Geometry check sheet. Reference: the model listing, model coordinates, mm. Face numbers are marked on the shaded views. A direction names the side the tool comes from. Give positions to 0.01 mm unless a question says otherwise; leave off trailing zeros. Loops run counter-clockwise (first coordinate to the right, second up) from the corner with the lowest first, then second, coordinate; pieces in that order, holes last. Notation, with made-up numbers: (16, -30.5) -> (35, -30.5) arc R22 ccw to (35, -13.5) -> close; hole circle Ø8 at (76, 73.5). An arc over 180 degrees is marked (long way). Write each question's results on one line, items separated by ' | '. Start each with the question number.
1) Scan lines: line 1 (Z direction, x = -30, y = -27.5); line 2 (Y direction, x = 2, z = 14); line 3 (Z direction, x = 26, y = -40.5). Record each from-to range of solid material in increasing order. Write a range as from..to.
2) Sectioned sample at B-B on x = 0. Record the cut outline in (y, z).
3) Depth check by flat-ended pin: pin 1 (4 mm diameter, centred on x = -23.81, z = 30.03, fed in from -Y); pin 2 (13.5 mm diameter, centred on x = -13.5, z = 31.5, fed in from +Y); pin 3 (8 mm diameter, centred on y = 6, z = 5, fed in from +X). Enter the tip coordinate at first touch or a pass-through.
4) Sectioned sample at D-D on z = 21.5. Record the cut outline in (x, y).
5) Sectioned sample at A-A on y = 12. Record the cut outline in (x, z), then the cut area to 3 significant figures.
6) Set-up check for the marked faces 1 and 2: record each of +Z, -Z, +X, -X, +Y, -Y from which the full face is reachable in a straight line by a thin tool's end or side.
7) Sectioned sample at C-C on y = -2.5. Record the cut outline in (x, z).
8) Draft check along X on the marked faces 3, 4 and 5. Enter one of: pulls with the +X half, pulls with the -X half, needs draft (parallel to the pull), parting line crosses it, or undercut.
```python
from build123d import *

# Parameters (mm, degrees)
F1_DEPTH = 13
F2_DEPTH = 40
F4_D     = 7


with BuildPart() as f1:
    # F0 (on Top) → F1 (new body)
    with BuildSketch(Plane.XY):
        with BuildLine():
            Line((30, 0), (35, 0))
            ThreePointArc((35, 0), (33.4744278282, 10.2206986834), (29.0307039098, 19.5504023104))
            add(Edge.make_bspline(
                [(29.0307039098, 19.5504023104), (27.7822040528, 21.275593448), (25.8954088148, 23.7212759458), (24.10664395, 23.9739441895)],
                knots=[0, 0, 0, 0, 0.5116358428, 0.5116358428, 0.5116358428, 0.5116358428], degree=3))
            Line((24.10664395, 23.9739441895), (23.5215793736, 23.9739441895))
            add(Edge.make_bspline(
                [(23.5215793736, 23.9739441895), (22.0865673396, 23.7581691141), (20.7707318469, 21.8685279115), (22.1448074946, 20.2387623393)],
                knots=[0.56784893, 0.56784893, 0.56784893, 0.56784893, 0.9854049804, 0.9854049804, 0.9854049804, 0.9854049804], degree=3))
            ThreePointArc((22.1448074946, 20.2387623393), (22.2219972589, 20.1539782134), (22.2988624189, 20.0688996914))
            ThreePointArc((22.2988624189, 20.0688996914), (28.0086225346, 10.7478864767), (30, 0))
        make_face()
        with BuildLine():
            Line((-35, -35), (0, -35))
            ThreePointArc((0, -35), (24.7487373415, -24.7487373415), (35, 0))
            Line((35, 0), (30, 0))
            ThreePointArc((30, 0), (0, -30), (-30, 0))
            ThreePointArc((-30, 0), (-28.0086225346, 10.7478864767), (-22.2988624189, 20.0688996914))
            ThreePointArc((-22.2988624189, 20.0688996914), (-22.2219972589, 20.1539782134), (-22.1448074946, 20.2387623393))
            add(Edge.make_bspline(
                [(-23.5215793736, 23.9739441895), (-22.0865673396, 23.7581691141), (-20.7707318469, 21.8685279115), (-22.1448074946, 20.2387623393)],
                knots=[0.56784893, 0.56784893, 0.56784893, 0.56784893, 0.9854049804, 0.9854049804, 0.9854049804, 0.9854049804], degree=3))
            Line((-23.5215793736, 23.9739441895), (-24.10664395, 23.9739441895))
            add(Edge.make_bspline(
                [(-29.0307039098, 19.5504023104), (-27.7822040528, 21.275593448), (-25.8954088148, 23.7212759458), (-24.10664395, 23.9739441895)],
                knots=[0, 0, 0, 0, 0.5116358428, 0.5116358428, 0.5116358428, 0.5116358428], degree=3))
            ThreePointArc((-29.0307039098, 19.5504023104), (-33.4744278282, 10.2206986834), (-35, 0))
            Line((-35, 0), (-35, -35))
        make_face()
        with BuildLine():
            ThreePointArc((35, 0), (24.7487373415, -24.7487373415), (0, -35))
            Line((0, -35), (35, -35))
            Line((35, -35), (35, 0))
        make_face()
        Polygon((35, -35), (0, -35), (-35, -35), (-35, -48), (35, -48), align=None)
    extrude(amount=F1_DEPTH)

    # F0 (on Top) → F2 (join)
    with BuildSketch(Plane.XY):
        Polygon((35, -35), (0, -35), (-35, -35), (-35, -48), (35, -48), align=None)
    extrude(amount=F2_DEPTH)

    # F4 (through all)
    with Locations(Plane(origin=(0, 0, 0), x_dir=(1, 0, 0), z_dir=(0, 1, 0))):
        with Locations((-23.8109529018, -30.0336983055), (23.8109529018, -30.0336983055)):
            Hole(F4_D / 2)


solid = f1.part
```
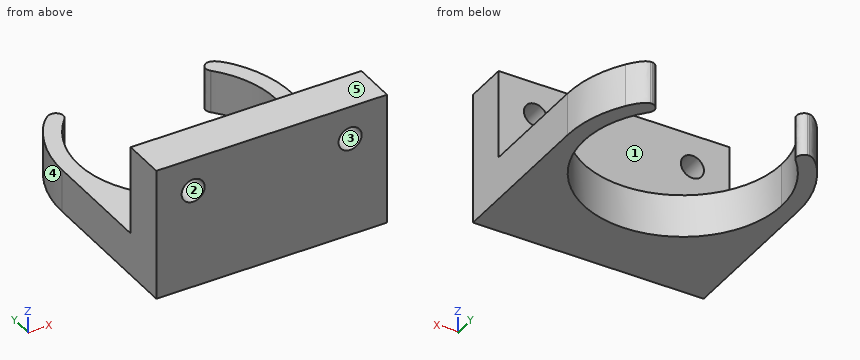
Result:
1) line 1: 0..13 | line 2: -48..-35 | line 3: 0..27.3, 32.76..40
2) outline: (-48, 0) -> (-30, 0) -> (-30, 13) -> (-35, 13) -> (-35, 40) -> (-48, 40) -> close
3) pin 1: through | pin 2: y = -35 | pin 3: x = 34.94
4) outline: (-35, -48) -> (35, -48) -> (35, -35) -> (-35, -35) -> close
5) outline: (-32.88, 0) -> (-27.5, 0) -> (-27.5, 13) -> (-32.88, 13) -> close; (27.5, 0) -> (32.88, 0) -> (32.88, 13) -> (27.5, 13) -> close | area: 140 mm^2
6) face 1: +Z, +X, -X, +Y | face 2: +Y, -Y
7) outline: (-35, 0) -> (-29.9, 0) -> (-29.9, 13) -> (-35, 13) -> close; (29.9, 0) -> (35, 0) -> (35, 13) -> (29.9, 13) -> close
8) face 3: undercut | face 4: pulls with the -X half | face 5: needs draft
